Check sheet for the drawn part. Datum: minimum x, y, z corner. Units: mm. Coordinates: 2 decimals unless noted, no trailing zeros. Write each loop counter-clockwise with the first axis right and the second up, starting at its lowest first coordinate (ties: lowest second). Pieces come first, ordered by that corner, then holes. Notation, with made-up numbers: M -27.75,-33 L -9.75,-33 A11 ccw -9.75,-20 Z; hole C -24.75,-28.75 d5. An arc over 180 degrees is marked long. Answer as CSV lines item,"result".
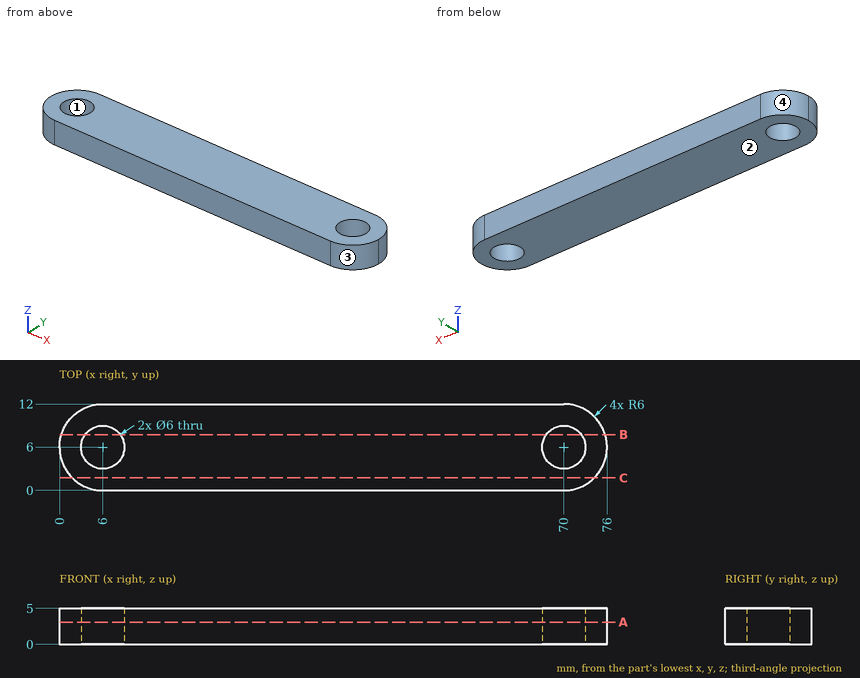
1) Depth check by flat-ended pin: P1, Ø2, axis at y = 3, z = 1.5, coming from the +X side. Enter the tip coordinate at first touch or a pass-through.
Answer key:
P1,"stops at x = 75.66"
2) Thickness scan on line 1 along Y through (x, z) = (70, 2.7); line 2 along X through (y, z) = (4, 0.4); line 3 along X through (y, z) = (2.5, 1.6). Record the ranges inside material, lowest first.
Answer key:
line 1,"y = 0 to 3, 9 to 12"
line 2,"x = 0.34 to 3.76, 8.24 to 67.76, 72.24 to 75.66"
line 3,"x = 1.13 to 74.87"
3) Section check A-A, the plane z = 3.1. Give the number of separate pieces and of enclosed holes in the cut face, plus the area to 3 significant figures.
Answer key:
separate pieces,"1"
enclosed holes,"2"
area,"825 mm2"
4) Section check C-C, the plane y = 1.75. Record the boundary of the cut face in (x, z).
Answer key:
outline,"M 1.76,0 L 74.24,0 L 74.24,5 L 1.76,5 Z"
5) Mould release check, pull along X, two halves, no side actions. Record for the marked faces 1, 2, 3 and 4: pulls with the +X half, pulls with the -X half, needs draft (parallel to the pull), parting line crosses it, or undercut.
Answer key:
face 1,"undercut"
face 2,"needs draft"
face 3,"pulls with the +X half"
face 4,"pulls with the -X half"
6) Section check B-B, the plane y = 7.75. Record the boundary of the cut face in (x, z).
Answer key:
outline,"M 0.26,0 L 3.56,0 L 3.56,5 L 0.26,5 Z; M 8.44,0 L 67.56,0 L 67.56,5 L 8.44,5 Z; M 72.44,0 L 75.74,0 L 75.74,5 L 72.44,5 Z"
